```python
from build123d import *

# Parameters (mm, degrees)
BOSS_EXTRUDE1_DEPTH = 6.88
SKETCH2_W           = 15
SKETCH2_H           = 6.858
CUT_EXTRUDE1_DEPTH  = 137.841297579
SKETCH3_R           = 3.25
CUT_EXTRUDE2_DEPTH  = 137.841297579
SKETCH4_R           = 1.1811
CUT_EXTRUDE3_DEPTH  = 137.841297579
CUT_EXTRUDE4_DEPTH  = 137.841297579
FILLET1_R           = 10
FILLET2_R           = 3
FILLET3_R           = 0.5
FILLET4_R           = 1
FILLET5_R           = 5.5512


with BuildPart() as part:
    # Sketch1 → Boss-Extrude1 (new body)
    with BuildSketch(Plane.XY):
        Polygon((-33.3545, 0), (0, 0), (0, -53.098), (-3.5, -53.098), (-3.5, -59.858), (0, -59.858), (0, -114.858), (-49.8185, -114.858), (-74.066498224, -62.858), (-33.899973056, -62.858), (-33.899973056, -59.858), (-30.899973056, -59.858), (-30.899973056, -53.098), (-37.999973056, -53.098), align=None)
    extrude(amount=BOSS_EXTRUDE1_DEPTH)

    # Sketch2 → Cut-Extrude1 (cut, through all)
    with BuildSketch(Plane.XY.offset(6.88)):
        with Locations((-20.7, -6.429)):
            Rectangle(SKETCH2_W, SKETCH2_H)
    extrude(amount=-CUT_EXTRUDE1_DEPTH, mode=Mode.SUBTRACT)

    # Sketch3 → Cut-Extrude2 (cut, through all)
    with BuildSketch(Plane.XY.offset(6.88)):
        with Locations((-15.75, -65.858)):
            Circle(SKETCH3_R)
        with Locations((-15.75, -105.858)):
            Circle(SKETCH3_R)
    extrude(amount=-CUT_EXTRUDE2_DEPTH, mode=Mode.SUBTRACT)

    # Sketch4 → Cut-Extrude3 (cut, through all)
    with BuildSketch(Plane.XY.offset(6.88)):
        with Locations((-46.5, -109.858)):
            Circle(SKETCH4_R)
        with Locations((-37.1528, -109.858)):
            Circle(SKETCH4_R)
        with BuildLine():
            Line((-27.95, -48.608), (-25.55, -48.608))
            ThreePointArc((-25.55, -48.608), (-24.8, -49.358), (-25.55, -50.108))
            Line((-25.55, -50.108), (-27.95, -50.108))
            ThreePointArc((-27.95, -50.108), (-28.7, -49.358), (-27.95, -48.608))
        make_face()
        with BuildLine():
            Line((-27.95, -41.608), (-25.55, -41.608))
            ThreePointArc((-25.55, -41.608), (-24.8, -42.358), (-25.55, -43.108))
            Line((-25.55, -43.108), (-27.95, -43.108))
            ThreePointArc((-27.95, -43.108), (-28.7, -42.358), (-27.95, -41.608))
        make_face()
    extrude(amount=-CUT_EXTRUDE3_DEPTH, mode=Mode.SUBTRACT)

    # Sketch5 → Cut-Extrude4 (cut, through all)
    with BuildSketch(Plane.XY.offset(6.88)):
        with BuildLine():
            Line((-15.725, -27.858), (-15.725, -35.858))
            ThreePointArc((-15.725, -35.858), (-17.5, -37.633), (-19.275, -35.858))
            Line((-19.275, -35.858), (-19.275, -27.858))
            ThreePointArc((-19.275, -27.858), (-17.5, -26.083), (-15.725, -27.858))
        make_face()
    extrude(amount=-CUT_EXTRUDE4_DEPTH, mode=Mode.SUBTRACT)

    # Fillet1
    fillet1_edges = [part.edges().sort_by_distance(p)[0] for p in [
        (0, -114.858, 3.44),
    ]]
    fillet(fillet1_edges, radius=FILLET1_R)

    # Fillet2
    fillet2_edges = [part.edges().sort_by_distance(p)[0] for p in [
        (-74.066498224, -62.858, 3.44),
        (-33.3545, 0, 3.44),
    ]]
    fillet(fillet2_edges, radius=FILLET2_R)

    # Fillet3
    fillet3_edges = [part.edges().sort_by_distance(p)[0] for p in [
        (0, -53.098, 3.44),
        (0, -59.858, 3.44),
        (-49.8185, -114.858, 3.44),
    ]]
    fillet(fillet3_edges, radius=FILLET3_R)

    # Fillet4
    fillet4_edges = [part.edges().sort_by_distance(p)[0] for p in [
        (0, 0, 3.44),
        (-37.999973056, -53.098, 3.44),
    ]]
    fillet(fillet4_edges, radius=FILLET4_R)

    # Fillet5
    # the kernel refuses this fillet: 5.5512 mm, written as the material it adds along each edge
    with BuildSketch(Plane(origin=(-33.899973056, -62.858, 0), x_dir=(0, 1, 0), z_dir=(0, 0, 1))) as fillet5_piece_1:
        with BuildLine():
            CenterArc((5.5512, 4.93023326), FILLET5_R, 180, 62.640229199)
            Line((0, 4.93023326), (-0.111024, 4.93023326))
            Line((-0.111024, 4.93023326), (-0.111024, 0))
            Line((-0.111024, 0), (0, -0.111024))
            ThreePointArc((0, -0.111024), (1.5, -0.111024), (2.948976, -0.098604665))
            Line((2.948976, -0.098604665), (3, 0))
        make_face()
    extrude(amount=6.88)


solid = part.part
```
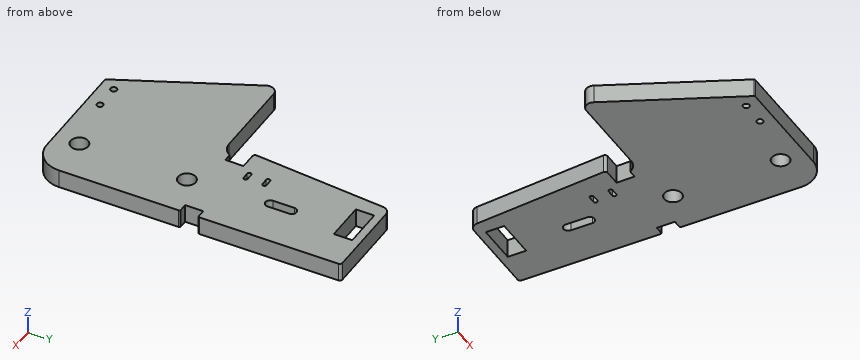
Geometry check sheet. Reference: the model listing, model coordinates, mm. Round coordinates to 2 decimals unless told otherwise and drop trailing zeros. Loops run counter-clockwise (first coordinate to the right, second up) from the corner with the lowest first, then second, coordinate; pieces in that order, holes last. Notation, with made-up numbers: (-10, 32.25) -> (11, 32.25) arc R22 cw to (11, 41.25) -> close; hole circle Ø9 at (9.5, -37.75). An arc over 180 degrees is marked (long way). Use a Markdown table: item, result.
(1) Go/stop test with flat-tipped pins: P1, Ø0.9, axis at x = -32.5, z = 4, coming from the +Y side; P2, Ø3.5, axis at x = -1.5, z = 2, coming from the -Y side; P3, Ø2, axis at y = -56, z = 2.5, coming from the -X side. Record where each tip stops, or that it passes through.
Calculated:
| item | result |
|---|---|
| P1 | y = -0.37 |
| P2 | y = -112.24 |
| P3 | x = -30.9 |
(2) Sectioned sample at B-B (x = -17.5). Enter the section's corners in (y, z), then the cut area to 3 significant figures.
Calculated:
| item | result |
|---|---|
| outline | (-114.86, 0) -> (-108.6, 0) -> (-108.6, 6.88) -> (-114.86, 6.88) -> close; (-103.12, 0) -> (-68.6, 0) -> (-68.6, 6.88) -> (-103.12, 6.88) -> close; (-63.12, 0) -> (-37.63, 0) -> (-37.63, 6.88) -> (-63.12, 6.88) -> close; (-26.08, 0) -> (-9.86, 0) -> (-9.86, 6.88) -> (-26.08, 6.88) -> close; (-3, 0) -> (0, 0) -> (0, 6.88) -> (-3, 6.88) -> close |
| area | 588 mm² |
(3) Sectioned sample at A-A (x = -46.5). Enter the section's corners in (y, z).
Calculated:
| item | result |
|---|---|
| outline | (-114.86, 0) -> (-111.04, 0) -> (-111.04, 6.88) -> (-114.86, 6.88) -> close; (-108.68, 0) -> (-62.86, 0) -> (-62.86, 6.88) -> (-108.68, 6.88) -> close |
(4) Sectioned sample at D-D (x = -54.5). Enter the section's corners in (y, z).
Calculated:
| item | result |
|---|---|
| outline | (-104.82, 0) -> (-62.86, 0) -> (-62.86, 6.88) -> (-104.82, 6.88) -> close |
(5) Sectioned sample at C-C (y = -82). Enter the section's corners in (x, z).
Calculated:
| item | result |
|---|---|
| outline | (-65.14, 0) -> (0, 0) -> (0, 6.88) -> (-65.14, 6.88) -> close |
(6) Scan lines: probe 1 along Y at (x, z) = (-28, 5.75); probe 2 along Y at (x, z) = (-46.5, 3.75); probe 3 along X at (y, z) = (-28.5, 6.5) (3 decimals). Record each from-to range of solid material in increasing order.
Calculated:
| item | result |
|---|---|
| probe 1 | -114.86 to -50.11, -48.61 to -43.11, -41.61 to -9.86, -3 to 0 |
| probe 2 | -114.86 to -111.04, -108.68 to -62.86 |
| probe 3 | -35.848 to -19.275, -15.725 to 0 |
